Design review of the part shown in the three views and the two pictorial views. Dimensions are in mm from the part's minimum x, y and z. Give positions to 0.01 mm unless a question says otherwise; leave off trailing zeros. Loops run counter-clockwise (first coordinate to the right, second up) from the corner with the lowest first, then second, coordinate; pieces in that order, holes last. Notation, with made-up numbers: (10, 74.5) - (48, 74.5) arc R23 cw to (48, 112.5) - close; hole circle Ø5 at (52, 83.5). An arc over 180 degrees is marked (long way). Answer in a Markdown table with one row per item.
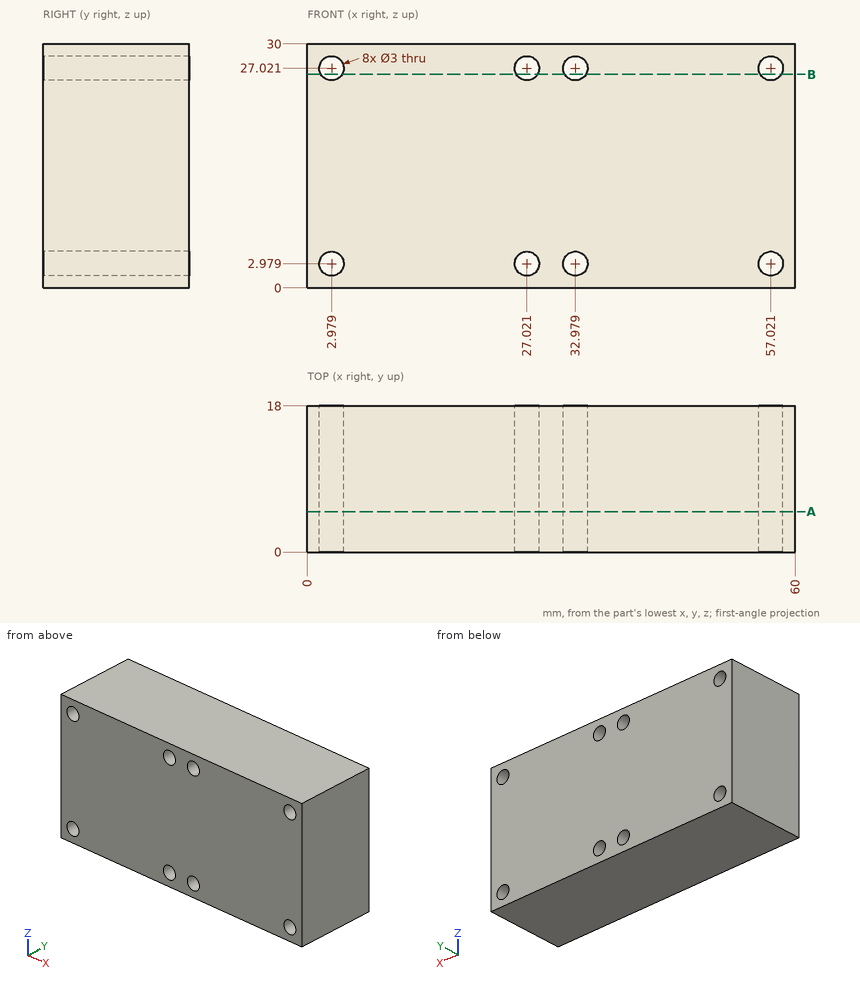
1. We need section A-A, the plane y = 5. Count the separate pieces of the cut face and the enclosed holes in it, and give its area (3 significant figures).
Values:
| item | result |
|---|---|
| separate pieces | 1 |
| enclosed holes | 8 |
| area | 1,740 mm^2 |
2. Wall thickness on line 1 (Z direction, x = 3, y = 1.5); line 2 (Z direction, x = 26, y = 10.25): over which ranges is each line inside the solid? List them lowest first. Write a range as [from, to].
Values:
| item | result |
|---|---|
| line 1 | z = [0, 1.48], [4.48, 25.52], [28.52, 30] |
| line 2 | z = [0, 1.88], [4.08, 25.92], [28.12, 30] |
3. We need section B-B, the plane z = 26.25. Give the boundary of the cut face in (x, y), and give its area (3 significant figures).
Values:
| item | result |
|---|---|
| outline | (0, 0) - (1.69, 0) - (1.69, 18) - (0, 18) - close; (4.27, 0) - (25.73, 0) - (25.73, 18) - (4.27, 18) - close; (28.31, 0) - (31.69, 0) - (31.69, 18) - (28.31, 18) - close; (34.27, 0) - (55.73, 0) - (55.73, 18) - (34.27, 18) - close; (58.31, 0) - (60, 0) - (60, 18) - (58.31, 18) - close |
| area | 895 mm^2 |
